Could you check a few things on this model? Use its own coordinates, in mm. A direction names the side the tool comes from. Give positions to 0.01 mm unless a question says otherwise; leave off trailing zeros. Loops run counter-clockwise (first coordinate to the right, second up) from the corner with the lowest first, then second, coordinate; pieces in that order, holes last.
1. I need wall thicknesses on line 1 along Y through (x, z) = (130.5, -223); line 2 along Z through (x, y) = (-216, 505); line 3 along Z through (x, y) = (-245, -19). Which ranges of each line are inside material? Lowest first, please.
2. For P1, Ø18, axis at x = 347, z = -40, coming from the +Y side; P2, Ø22.5, axis at x = 136.6, z = -255, coming from the -Y side; P3, Ø10, axis at x = 109, y = -7.5, coming from the -Z side, each with a flat end and sliding along its axis, tell me the tip position at first contact or that it passes through.
3. Imagine slicing it at B-B (x = 191). List the corners of the cut face in (y, z) for me, plus the area to 3 significant figures.
4. For faces 1 (the flat face through (319, -111, -180)), 2 (the flat face through (-230, -111, -155)), 3 (the flat face through (-230, -12, -210)), 4 (the flat face through (50.286, -12.325, -240.42)), 5 (the flat face through (332, -111, -155)), which set-ups out of +Z, -Z, +X, -X, +Y, -Y let a thin tool reach every point of the face, with its end or its side?
5. Imagine slicing it at A-A (y = 42). List the corners of the cut face in (x, z) for me.
6. Thinking about a two-plate mould opening in X: for faces 6 (the flat face through (319, -200, -154)), 7 (the flat face through (148.05, -12.32, -229.77)), 8 (the cylindrical face through (138.99, -6.41, -264.71)), which applies, +X half, -X half, draft (parallel to the pull), parting line (faces both ways), or undercut?
```python
from build123d import *

# Parameters (mm, degrees)
F0_R          = 7
F0_R_2        = 6.5
F1_DEPTH      = 25
F2_W          = 25.4
F2_H          = 50.8
F3_DEPTH      = 200
F3_DEPTH_BACK = 600
F6_DEPTH      = 65
F8_R          = 15
F8_R_2        = 7
F9_DEPTH      = 10
F10_R         = 15
F10_R_2       = 7
F11_DEPTH     = 10
F12_R         = 7.5
F13_REACH     = 111.2142034356
F14_R         = 10
F14_R_2       = 7
F15_DEPTH     = 12.7
F16_R         = 10
F16_R_2       = 7
F17_DEPTH     = 12.7


with BuildPart() as f1:
    # F0 (on Front) → F1 (new body)
    with BuildSketch(Plane.XZ):
        with BuildLine():
            Line((-230, 0), (-301.7204504189, 102.2319018363))
            ThreePointArc((-301.7204504189, 102.2319018363), (-322.6146771319, 105.8967742855), (-326.2795495811, 85.0025475726))
            Line((-326.2795495811, 85.0025475726), (-260, -9.4737749679))
            Line((-260, -9.4737749679), (-260, -270))
            Line((-260, -270), (0, -270))
            Line((0, -270), (102, -210))
            Line((102, -210), (121.6, -210))
            Line((121.6, -210), (128.6, -249))
            ThreePointArc((128.6, -249), (136.6, -265), (144.6, -249))
            Line((144.6, -249), (151.6, -210))
            Line((151.6, -210), (362, -210))
            Line((362, -210), (362, -9.4737749679))
            Line((362, -9.4737749679), (428.2795495811, 85.0025475726))
            ThreePointArc((428.2795495811, 85.0025475726), (424.6146771319, 105.8967742855), (403.7204504189, 102.2319018363))
            Line((403.7204504189, 102.2319018363), (332, 0))
            Line((332, 0), (332, -129.2))
            Line((332, -129.2), (332, -180))
            Line((332, -180), (306.6, -180))
            Line((306.6, -180), (102, -180))
            Line((102, -180), (0, -240))
            Line((0, -240), (-230, -240))
            Line((-230, -240), (-230, 0))
        make_face()
        with Locations((-60, -255)):
            Circle(F0_R, mode=Mode.SUBTRACT)
        with Locations((136.6, -255)):
            Circle(F0_R, mode=Mode.SUBTRACT)
        with Locations((-245, -40)):
            Circle(F0_R, mode=Mode.SUBTRACT)
        with Locations((-314, 93.6172247045)):
            Circle(F0_R_2, mode=Mode.SUBTRACT)
        with Locations((347, -40)):
            Circle(F0_R, mode=Mode.SUBTRACT)
        with Locations((416, 93.6172247045)):
            Circle(F0_R_2, mode=Mode.SUBTRACT)
    extrude(amount=F1_DEPTH)

    # F2 (on Front) → F3 (join, two sides)
    with BuildSketch(Plane.XZ) as f3_sk:
        with Locations((319.3, -154.6)):
            Rectangle(F2_W, F2_H)
        with Locations((-217.3, -154.6)):
            Rectangle(F2_W, F2_H)
    extrude(amount=F3_DEPTH)
    extrude(f3_sk.sketch, amount=-F3_DEPTH_BACK)

    # F5 (on face) → F6 (join)
    with BuildSketch(Plane.XY.offset(-129.2)):
        with BuildLine():
            ThreePointArc((316.7348489251, 413.4476946559), (314.9981767274, 400.2563596678), (326.8, 406.4))
            ThreePointArc((326.8, 406.4), (323.6018232726, 412.5436403322), (316.7348489251, 413.4476946559))
        make_face()
    extrude(amount=F6_DEPTH)

    # F8 (on face) → F9 (join, symmetric)
    with BuildSketch(Plane(origin=(412.5634376322, 150.1608110447, 0), x_dir=(0.3420201433, -0.9396926208, 0), z_dir=(-0.9396926208, -0.3420201433, 0))):
        with Locations((-272.6840493235, -64.6)):
            Circle(F8_R)
        with Locations((-272.6840493235, -64.6)):
            Circle(F8_R_2, mode=Mode.SUBTRACT)
    extrude(amount=F9_DEPTH, both=True)



with BuildPart() as f11:
    # F10 (on face) → F11 (new body, symmetric)
    with BuildSketch(Plane(origin=(412.5634376322, 150.1608110447, 0), x_dir=(0.3420201433, -0.9396926208, 0), z_dir=(-0.9396926208, -0.3420201433, 0))):
        with Locations((-272.6840493235, -240)):
            Circle(F10_R)
        with Locations((-272.6840493235, -240)):
            Circle(F10_R_2, mode=Mode.SUBTRACT)
    extrude(amount=F11_DEPTH, both=True)


with BuildPart() as f1_1:
    add(f1.part)

    add(f11.part)  # F13 merges F11
    f13_end = f1_1.faces().sort_by_distance((314.1696978501, 420.4953893118, -240))[0]
    # F12 (on face) → F13 (join, up to a face of the model that its end follows)
    with BuildSketch(Plane(origin=(0, 0, -180), x_dir=(1, 0, 0), z_dir=(0, 0, -1))):
        with Locations((319.3, -406.4)):
            Circle(F12_R)
    f13_long = extrude(amount=F13_REACH, mode=Mode.PRIVATE)
    add(split(f13_long, bisect_by=f13_end, keep=Keep.ALL, mode=Mode.PRIVATE).solids().sort_by_distance((319.3, 406.4, -180))[0])

    # F14 (on face) → F15 (join)
    with BuildSketch(Plane.XZ):
        with Locations((136.6, -255)):
            Circle(F14_R)
        with Locations((136.6, -255)):
            Circle(F14_R_2, mode=Mode.SUBTRACT)
    extrude(amount=-F15_DEPTH)

    # F16 (on face) → F17 (join)
    with BuildSketch(Plane.XZ):
        with Locations((347, -40)):
            Circle(F16_R)
        with Locations((347, -40)):
            Circle(F16_R_2, mode=Mode.SUBTRACT)
    extrude(amount=-F17_DEPTH)


solid = f1_1.part
```
Derived:
1. line 1: y = -25 to 0
1. line 2: z = -180 to -129.2
1. line 3: z = -270 to -47, -33 to 21.38
2. P1: stops at y = 12.7
2. P2: stops at y = -25
2. P3: stops at z = -210
3. outline: (-25, -210) - (0, -210) - (0, -180) - (-25, -180) - close
3. area: 750 mm2
4. face 1: -Z, +X, -X, -Y
4. face 2: +Z, -Z, -X, -Y
4. face 3: +Y, -Y
4. face 4: -Z, +Y, -Y
4. face 5: +Z, -Z, +X, -Y
5. outline: (-230, -180) - (-204.6, -180) - (-204.6, -129.2) - (-230, -129.2) - close; (306.6, -180) - (332, -180) - (332, -129.2) - (306.6, -129.2) - close
6. face 6: draft
6. face 7: +X half
6. face 8: undercut
